CAD build for the part. Positions are in the model's coordinates, mm. A direction names the side the tool comes from. Give positions to 0.01 mm unless a question says otherwise; leave off trailing zeros. Order: outer loops, then holes, each group sorted by start corner. A loop starts at its lowest first (then second) coordinate and runs counter-clockwise, first axis right, second up.
Item 1: Two-plate mould, pull along X, no slides. Class faces 6 (the flat face through (-15.75, 1, 0)), 7 (the flat face through (12, 0, 16)), 8 (the flat face through (-11, -3, 15)), 9 (the cylindrical face through (13.8, 2.04, -17.63)): released by +X, released by -X, zero draft, split by the parting line, or undercut.
Item 2: Wall check: L1, parallel to X at y = -1.65, z = 15.9; L2, parallel to Y at x = 12, z = -1; L3, parallel to Y at x = 4, z = 18.5. Give the ranges that are in metal, low to high.
Item 3: Which spindle directions (+Z, -Z, +X, -X, +Y, -Y) get a long thin tool onto all of the face, cutting with end or side? Do faces 1 (the flat face through (15.45, 2, 0)), 2 (the flat face through (0, 2, 19.2)), 3 (the cylindrical face through (11.384, -1.479, -17.747)), 4 (the cylindrical face through (-13.88, 2.04, -17.55)), 5 (the flat face through (-15.45, 2, 0)). Say none if no direction does.
Item 4: Band-saw the part on A-A on y = 0.8. Give the cut face in (x, z), plus the area to 3 significant figures.
Item 5: Band-saw the part on D-D on z = 2.5. Give the cut face in (x, y) (3 decimals), plus the area to 3 significant figures.
Item 6: Flat gauge pins, fed straight in: P1, Ø0.6, axis at x = 12, z = 16, coming from the -Y side; P2, Ø0.7, axis at x = 0.5, y = 2, coming from the -Z side; P3, Ø1.6, axis at x = -12.15, z = 15.9, coming from the +Y side. Where does each tip first touch, or does it go through?
Item 7: Band-saw the part on C-C on z = -15.9. Give the cut face in (x, y), plus the area to 3 significant figures.
Item 8: Band-saw the part on B-B on x = 4. Give the cut face in (y, z), plus the area to 3 significant figures.
```python
from build123d import *

# Parameters (mm, degrees)
EXTRUDE_1_DEPTH = 1.6
EXTRUDE_2_DEPTH = 1
EXTRUDE_3_DEPTH = 0.9
SKETCH_4_R      = 2
SKETCH_4_R_2    = 1
EXTRUDE_4_DEPTH = 3


with BuildPart() as part:
    # 草图1 → 凸台-拉伸1 (new body)
    with BuildSketch(Plane(origin=(0, 0, 0), x_dir=(1, 0, 0), z_dir=(0, 1, 0))):
        with BuildLine():
            Line((-10.25, 19.5), (10.25, 19.5))
            ThreePointArc((10.25, 19.5), (14.139087297, 17.889087297), (15.75, 14))
            Line((15.75, 14), (15.75, -14.5))
            ThreePointArc((15.75, -14.5), (14.285533906, -18.035533906), (10.75, -19.5))
            Line((10.75, -19.5), (-10.75, -19.5))
            ThreePointArc((-10.75, -19.5), (-14.285533906, -18.035533906), (-15.75, -14.5))
            Line((-15.75, -14.5), (-15.75, 14))
            ThreePointArc((-15.75, 14), (-14.139087297, 17.889087297), (-10.25, 19.5))
        make_face()
    extrude(amount=EXTRUDE_1_DEPTH)

    # 草图2 → 凸台-拉伸2 (add)
    with BuildSketch(Plane(origin=(0, 1.6, 0), x_dir=(1, 0, 0), z_dir=(0, 1, 0))):
        with BuildLine():
            Line((-8.985, 17.58), (8.985, 17.58))
            ThreePointArc((8.985, 17.58), (12.520533906, 16.115533906), (13.985, 12.58))
            Line((13.985, 12.58), (13.985, -10.05))
            ThreePointArc((13.985, -10.05), (12.520533906, -13.585533906), (8.985, -15.05))
            Line((8.985, -15.05), (-8.985, -15.05))
            ThreePointArc((-8.985, -15.05), (-12.520533906, -13.585533906), (-13.985, -10.05))
            Line((-13.985, -10.05), (-13.985, 12.58))
            ThreePointArc((-13.985, 12.58), (-12.520533906, 16.115533906), (-8.985, 17.58))
        make_face()
    extrude(amount=EXTRUDE_2_DEPTH)

    # 草图3 → 凸台-拉伸3 (add)
    with BuildSketch(Plane(origin=(0, 1.6, 0), x_dir=(1, 0, 0), z_dir=(0, 1, 0))):
        with BuildLine():
            Line((-9.95, 19.2), (9.95, 19.2))
            ThreePointArc((9.95, 19.2), (13.839087297, 17.589087297), (15.45, 13.7))
            Line((15.45, 13.7), (15.45, -14.2))
            ThreePointArc((15.45, -14.2), (13.985533906, -17.735533906), (10.45, -19.2))
            Line((10.45, -19.2), (-10.45, -19.2))
            ThreePointArc((-10.45, -19.2), (-13.985533906, -17.735533906), (-15.45, -14.2))
            Line((-15.45, -14.2), (-15.45, 13.7))
            ThreePointArc((-15.45, 13.7), (-13.839087297, 17.589087297), (-9.95, 19.2))
        make_face()
    extrude(amount=EXTRUDE_3_DEPTH)

    # 草图4 → 凸台-拉伸4 (add)
    # profile 1 of 4: a face of its own
    with BuildSketch(Plane.XZ):
        with Locations(Location((-12.15, 15.9, 0), (0, 0, 270))):
            Circle(SKETCH_4_R)
        with Locations(Location((-12.15, 15.9, 0), (0, 0, 270))):
            Circle(SKETCH_4_R_2, mode=Mode.SUBTRACT)
    # profile 2 of 4: a face of its own
    with BuildSketch(Plane.XZ):
        with Locations(Location((12.15, 15.9, 0), (0, 0, 270))):
            Circle(SKETCH_4_R)
        with Locations(Location((12.15, 15.9, 0), (0, 0, 270))):
            Circle(SKETCH_4_R_2, mode=Mode.SUBTRACT)
    # profile 3 of 4: a face of its own
    with BuildSketch(Plane.XZ):
        with Locations(Location((12.15, -15.9, 0), (0, 0, 270))):
            Circle(SKETCH_4_R)
        with Locations(Location((12.15, -15.9, 0), (0, 0, 270))):
            Circle(SKETCH_4_R_2, mode=Mode.SUBTRACT)
    # profile 4 of 4: a face of its own
    with BuildSketch(Plane.XZ):
        with Locations(Location((-12.15, -15.9, 0), (0, 0, 270))):
            Circle(SKETCH_4_R)
        with Locations(Location((-12.15, -15.9, 0), (0, 0, 270))):
            Circle(SKETCH_4_R_2, mode=Mode.SUBTRACT)
    extrude(amount=EXTRUDE_4_DEPTH)


solid = part.part
```
The answers:
1. face 6: released by -X
1. face 7: undercut
1. face 8: zero draft
1. face 9: released by +X
2. L1: x = -14.15 to -13.15, -11.15 to -10.15, 10.15 to 11.15, 13.15 to 14.15
2. L2: y = 0 to 2.6
2. L3: y = 0 to 2.5
3. face 1: +Z, -Z, +X, +Y
3. face 2: +Z, +X, -X, +Y
3. face 3: -Y
3. face 4: -Z, -X, +Y
3. face 5: +Z, -Z, -X, +Y
4. outline: (-15.75, -14) arc R5.5 ccw to (-10.25, -19.5) - (10.25, -19.5) arc R5.5 ccw to (15.75, -14) - (15.75, 14.5) arc R5 ccw to (10.75, 19.5) - (-10.75, 19.5) arc R5 ccw to (-15.75, 14.5) - close
4. area: 1,200 mm2
5. outline: (-15.75, 0) - (15.75, 0) - (15.75, 1.6) - (15.45, 1.6) - (15.45, 2.5) - (13.985, 2.5) - (13.985, 2.6) - (-13.985, 2.6) - (-13.985, 2.5) - (-15.45, 2.5) - (-15.45, 1.6) - (-15.75, 1.6) - close
5. area: 81.0 mm2
6. P1: stops at y = 0
6. P2: stops at z = -19.2
6. P3: stops at y = 2.5
7. outline: (-15.41, 0) - (-14.15, 0) - (-14.15, -3) - (-13.15, -3) - (-13.15, 0) - (-11.15, 0) - (-11.15, -3) - (-10.15, -3) - (-10.15, 0) - (10.15, 0) - (10.15, -3) - (11.15, -3) - (11.15, 0) - (13.15, 0) - (13.15, -3) - (14.15, -3) - (14.15, 0) - (15.41, 0) - (15.41, 1.6) - (14.99, 1.6) - (14.99, 2.5) - (12.72, 2.5) - (12.72, 2.6) - (-12.72, 2.6) - (-12.72, 2.5) - (-14.99, 2.5) - (-14.99, 1.6) - (-15.41, 1.6) - close
7. area: 90.8 mm2
8. outline: (0, -19.5) - (1.6, -19.5) - (1.6, -19.2) - (2.5, -19.2) - (2.5, -17.58) - (2.6, -17.58) - (2.6, 15.05) - (2.5, 15.05) - (2.5, 19.2) - (1.6, 19.2) - (1.6, 19.5) - (0, 19.5) - close
8. area: 100 mm2
